Here's how the part is built. I have some questions about the finished solid (model axes, mm). Face numbers are marked on the shaded views. A direction names the side the tool comes from. Coordinates: 2 decimals unless noted, no trailing zeros. Order: outer loops, then holes, each group sorted by start corner. A loop starts at its lowest first (then second) coordinate and runs counter-clockwise, first axis right, second up. Notation, with made-up numbers: (79.5, 69.25) - (122.5, 69.25) arc R10 cw to (122.5, 81.25) - close; hole circle Ø4 at (28.25, 33.5). An arc over 180 degrees is marked (long way). Answer as CSV lines item,"result". Start each with the question number.
Item 1: We'd pull the mould along X, two halves only. Please class the marked faces 4, 5 and 6: pulls with the +X half, pulls with the -X half, needs draft (parallel to the pull), parting line crosses it, or undercut.
Item 2: Imagine slicing it at A-A on z = 0. List the corners of the cut face in (x, y) for me.
Item 3: I'm going to push flat-ended pins straight in: pin 1 (4.5 mm diameter, centred on x = 7, z = -2, fed in from +Y); pin 2 (0.9 mm diameter, centred on y = -2, z = 2.5, fed in from +X); pin 3 (1.5 mm diameter, centred on y = -7.5, z = -8, fed in from -X). Where does each tip first touch, or does it pass through?
Item 4: Imagine slicing it at B-B on x = 0. List the corners of the cut face in (y, z) for me, and give its area (3 significant figures).
Item 5: Imagine slicing it at D-D on z = 3.75. List the corners of the cut face in (x, y) for me.
Item 6: Imagine slicing it at C-C on y = -2.5. List the corners of the cut face in (x, z) for me.
Item 7: On a 3-axis mill with a long thin cutter (end or side, diameter ignored), from which of +Z, -Z, +X, -X, +Y, -Y can I reach the whole of each face in a straight line? I mean the marked faces 1, 2 and 3. Say none if no direction works.
Item 8: I need wall thicknesses on line 1 (X direction, y = -3.5, z = 0); line 2 (Z direction, x = 0, y = -6). Which ranges of each line are inside material? Lowest first, please.
from build123d import *

# Parameters (mm, degrees)
EXTRUDE_1_DEPTH = 10
FILLET_1_R      = 0.2


with BuildPart() as part:
    # Эскиз1 → Бобышка-Вытянуть1 (new body, symmetric)
    with BuildSketch(Plane.XY):
        Polygon((4, 0), (-4, 0), (-4, -3.3), (-9.75, -3.3), (-9.75, -5.8), (-4, -9.5), (4, -9.5), (9.75, -5.8), (9.75, -3.3), (4, -3.3), align=None)
    extrude(amount=EXTRUDE_1_DEPTH, both=True)

    # Эскиз4 → Отверстие обработанное метчиком M43 (revolve, cut)
    with BuildSketch(Plane(origin=(0, 0, 0), x_dir=(0, 0, 1), z_dir=(1, 0, 0))):
        Polygon((0, 0), (0, 9.5), (2.15, 9.5), (1.65, 9), (1.65, 0.5), (2.15, 0), align=None)
    revolve(axis=Axis((0, 6.35, 0), (0, -1, 0)), mode=Mode.SUBTRACT)

    # Скругление1
    fillet_1_edges = [part.edges().sort_by_distance(p)[0] for p in [
        (-4, 0, 0),
        (4, 0, 0),
        (4, -3.3, 0),
        (9.75, -3.3, 0),
        (4, -9.5, 0),
        (-4, -9.5, 0),
        (-9.75, -3.3, 0),
        (-4, -3.3, 0),
    ]]
    fillet(fillet_1_edges, radius=FILLET_1_R)


solid = part.part
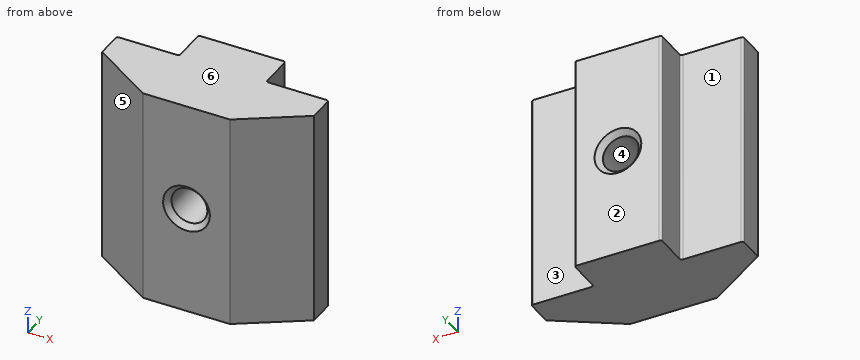
Responses:
1,face 4,"undercut"
1,face 5,"pulls with the -X half"
1,face 6,"needs draft"
2,outline,"(-9.75, -5.8) - (-4.05, -9.47) arc R0.2 ccw to (-3.94, -9.5) - (-2.15, -9.5) - (-1.65, -9) - (-1.65, -0.5) - (-2.15, 0) - (-3.8, 0) arc R0.2 ccw to (-4, -0.2) - (-4, -3.1) arc R0.2 cw to (-4.2, -3.3) - (-9.55, -3.3) arc R0.2 ccw to (-9.75, -3.5) - close; (1.65, -9) - (2.15, -9.5) - (3.94, -9.5) arc R0.2 ccw to (4.05, -9.47) - (9.75, -5.8) - (9.75, -3.5) arc R0.2 ccw to (9.55, -3.3) - (4.2, -3.3) arc R0.2 cw to (4, -3.1) - (4, -0.2) arc R0.2 ccw to (3.8, 0) - (2.15, 0) - (1.65, -0.5) - close"
3,pin 1,"stops at y = -3.3"
3,pin 2,"stops at x = 4"
3,pin 3,"stops at x = -8.27"
4,outline,"(-9.5, -10) - (0, -10) - (0, -2.15) - (-0.5, -1.65) - (-9, -1.65) - (-9.5, -2.15) - close; (-9.5, 2.15) - (-9, 1.65) - (-0.5, 1.65) - (0, 2.15) - (0, 10) - (-9.5, 10) - close"
4,area,"158 mm^2"
5,outline,"(-9.75, -5.8) - (-4.05, -9.47) arc R0.2 ccw to (-3.94, -9.5) - (3.94, -9.5) arc R0.2 ccw to (4.05, -9.47) - (9.75, -5.8) - (9.75, -3.5) arc R0.2 ccw to (9.55, -3.3) - (4.2, -3.3) arc R0.2 cw to (4, -3.1) - (4, -0.2) arc R0.2 ccw to (3.8, 0) - (-3.8, 0) arc R0.2 ccw to (-4, -0.2) - (-4, -3.1) arc R0.2 cw to (-4.2, -3.3) - (-9.55, -3.3) arc R0.2 ccw to (-9.75, -3.5) - close"
6,outline,"(-4, -10) - (4, -10) - (4, 10) - (-4, 10) - close; hole circle Ø3.3 at (0, 0)"
7,face 1,"+Z, -Z, -X, +Y"
7,face 2,"+Z, -Z, +X, -X, +Y"
7,face 3,"+Z, -Z, +X, +Y"
8,line 1,"x = -9.75 to -1.65, 1.65 to 9.75"
8,line 2,"z = -10 to -1.65, 1.65 to 10"
